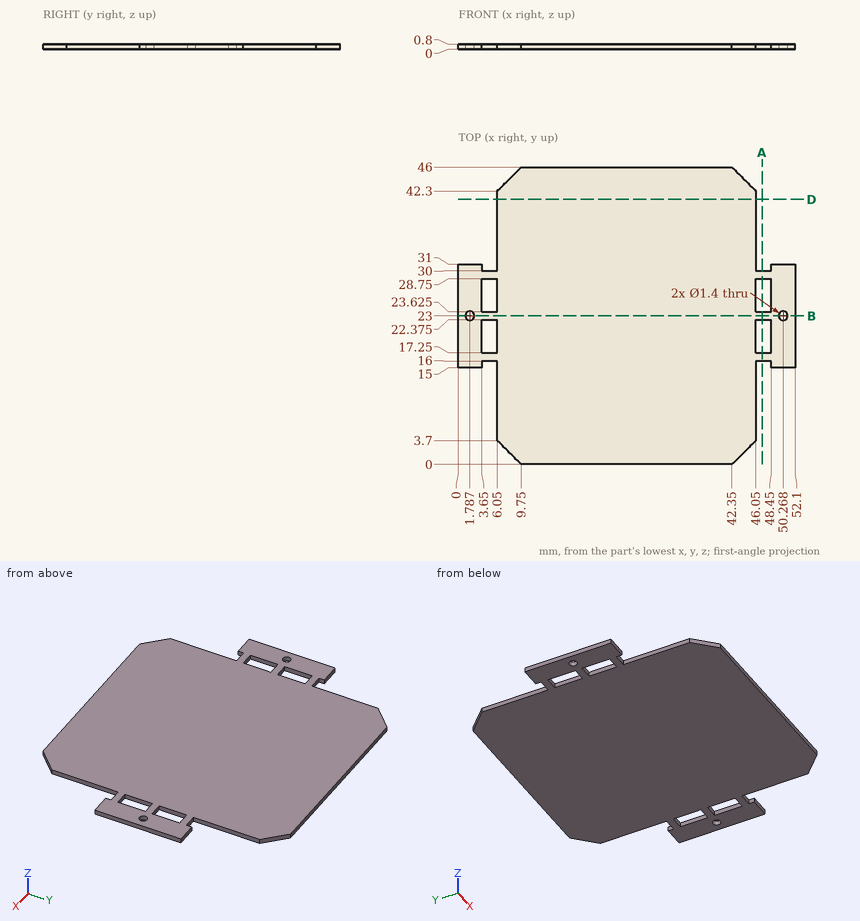
The figure shows three views and two pictorial views of one solid part (mm, origin at its lowest corner). Answer the questions. Give positions to 0.01 mm unless a question says otherwise; leave off trailing zeros. Write each loop counter-clockwise with the first axis right and the second up, starting at its lowest first coordinate (ties: lowest second). Pieces come first, ordered by that corner, then holes. Notation, with made-up numbers: (18.25, 0.25) - (35.25, 0.25) arc R16 ccw to (35.25, 19.25) - close; hole circle Ø1 at (36, -28). An arc over 180 degrees is marked (long way). Return JSON: item names as keys, results as strings.
Q1. A cutting plane is placed at A-A, the plane x = 47. Count the separate pieces of the cut face and the enclosed holes in it.
Reply:
{"separate pieces": "3", "enclosed holes": "0"}
Q2. A cutting plane is placed at D-D, the plane y = 41. Determine the outline of the cut face in (x, z).
Reply:
{"outline": "(6.05, 0) - (46.05, 0) - (46.05, 0.8) - (6.05, 0.8) - close"}
Q3. A cutting plane is placed at B-B, the plane y = 23. Determine the outline of the cut face in (x, z).
Reply:
{"outline": "(0, 0) - (1.09, 0) - (1.09, 0.8) - (0, 0.8) - close; (2.49, 0) - (49.57, 0) - (49.57, 0.8) - (2.49, 0.8) - close; (50.97, 0) - (52.1, 0) - (52.1, 0.8) - (50.97, 0.8) - close"}
Q4. Consider line 1 along X through (y, z) = (25, 0.55); line 2 along X through (y, z) = (13, 0.75); line 3 along Y through (x, z) = (9, 0.5). Determine where each line is inside the solid, lowest interval first. Write a range as [from, to].
Reply:
{"line 1": "[0, 3.65], [6.05, 46.05], [48.45, 52.1]", "line 2": "[6.05, 46.05]", "line 3": "[0.75, 45.25]"}
Q5. Given P1, Ø1.5, axis at x = 16, y = 7, coming from the -Z side, flat-ended and moving along its own axis, determine where the tip first touches the part or whether it passes through.
Reply:
{"P1": "z = 0"}
